Answer from the drawing. Dimensions are ordinates in mm from the lowest x, y and z of the part. A direction names the side the tool comes from. Give positions to 0.01 mm unless a question says otherwise; leave off trailing zeros. Loops run counter-clockwise (first coordinate to the right, second up) from the corner with the lowest first, then second, coordinate; pieces in that order, holes last.
(1) Find section B-B, the plane x = 99. Write down the section's boundary in (y, z), then the cut area to 4 significant figures.
(2) Each of these flat-tipped pins is pushed along its axis until it touches: P1, Ø6, axis at y = 20.5, z = 83, coming from the -X side; P2, Ø1, axis at x = 53.5, y = 6, coming from the +Z side; P3, Ø4, axis at y = 14, z = 43, coming from the -X side. Where does it stop, or does it pass through?
(3) Which of the six approach directions +Z, -Z, +X, -X, +Y, -Y give full straight-line access (tool end or side, diameter ignored) to the marked faces 1 and 2?
(4) Find section C-C, the plane z = 35. Write down the section's boundary in (x, y).
(5) Find section A-A, the plane y = 10. Write down the section's boundary in (x, z), then the cut area to 3 significant figures.
(6) Straight lines are drawn through the part: probe 1 along X at (y, z) = (19, 99.5); probe 2 along X at (y, z) = (11.75, 63); probe 3 along Z at (x, y) = (8, 11.5). For each, find the intervals that lie inside material, in ascending order.
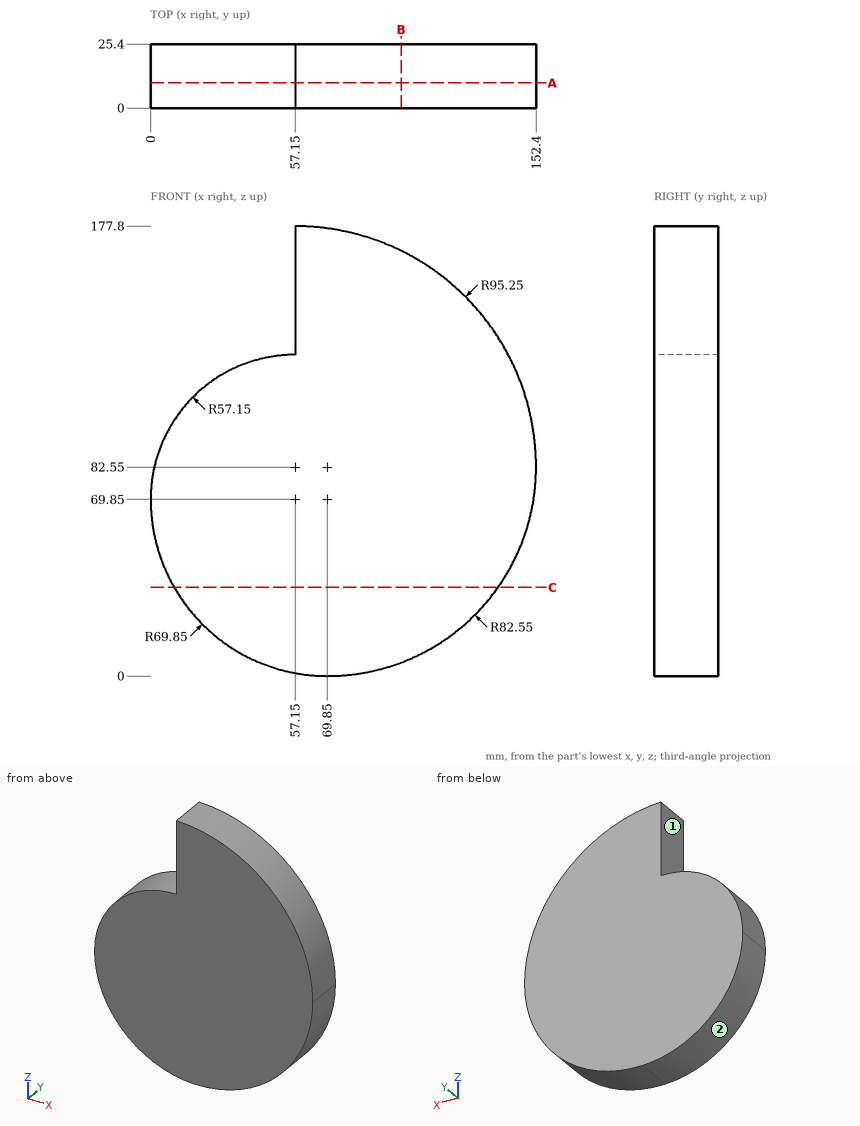
Entries:
1. outline: (0, 5.32) - (25.4, 5.32) - (25.4, 168.11) - (0, 168.11) - close
1. area: 4,135 mm2
2. P1: stops at x = 0.91
2. P2: stops at z = 126.91
2. P3: stops at x = 4.57
3. face 1: +Z, -X, +Y, -Y
3. face 2: -Z, -X, +Y, -Y
4. outline: (9.31, 0) - (137.33, 0) - (137.33, 25.4) - (9.31, 25.4) - close
5. outline: (0, 69.85) arc R69.85 ccw to (69.85, 0) arc R82.55 ccw to (152.4, 82.55) arc R95.25 ccw to (57.15, 177.8) - (57.15, 127) arc R57.15 ccw to start
5. area: 19,000 mm2
6. probe 1: x = 8.29 to 150.88
6. probe 2: x = 0.34 to 150.05
6. probe 3: z = 37.39 to 99.01
